from build123d import *

# Parameters (mm, degrees)
BOSS_EXTRUDE1_DEPTH = 1.2
SKETCH1_4_W         = 11
SKETCH1_4_H         = 2.5
BOSS_EXTRUDE2_DEPTH = 1.2
CUT_EXTRUDE1_DEPTH  = 14.654303351
SKETCH4_R           = 6.05
SKETCH4_R_2         = 2.55
CUT_EXTRUDE3_DEPTH  = 0.2


with BuildPart() as part:
    # Sketch1 → Boss-Extrude1 (new body)
    with BuildSketch(Plane(origin=(0, 0, 0), x_dir=(1, 0, 0), z_dir=(0, 1, 0))):
        with BuildLine():
            Line((-5.5, 0), (-1.5, 0))
            ThreePointArc((-1.5, 0), (0, 1.5), (1.5, 0))
            Line((1.5, 0), (5.5, 0))
            Line((5.5, 0), (5.5, 5.5))
            Line((5.5, 5.5), (-5.5, 5.5))
            Line((-5.5, 5.5), (-5.5, 0))
        make_face()
        with BuildLine():
            ThreePointArc((1.5, 0), (0, -1.5), (-1.5, 0))
            Line((-1.5, 0), (-5.5, 0))
            Line((-5.5, 0), (-5.5, -5.5))
            Line((-5.5, -5.5), (5.5, -5.5))
            Line((5.5, -5.5), (5.5, 0))
            Line((5.5, 0), (1.5, 0))
        make_face()
    extrude(amount=BOSS_EXTRUDE1_DEPTH)

    # Sketch1_4 → Boss-Extrude2 (add)
    with BuildSketch(Plane(origin=(0, 0, 0), x_dir=(1, 0, 0), z_dir=(0, 1, 0))):
        with Locations((0, 6.75)):
            Rectangle(SKETCH1_4_W, SKETCH1_4_H)
    extrude(amount=BOSS_EXTRUDE2_DEPTH)

    # Sketch3 → Cut-Extrude1 (cut, through all)
    with BuildSketch(Plane(origin=(5.5, 0, 0), x_dir=(0, 0, -1), z_dir=(1, 0, 0))):
        with BuildLine():
            Line((8, 1.2), (5.5, 1.2))
            add(Edge.make_bspline(
                [(5.5, 1.2), (6.993685342, 0.880481124), (8, 0)],
                knots=[0, 0, 0, 0.506360877, 0.506360877, 0.506360877], degree=2))
            Line((8, 0), (8, 1.2))
        make_face()
    extrude(amount=-CUT_EXTRUDE1_DEPTH, mode=Mode.SUBTRACT)

    # Sketch4 → Cut-Extrude3 (cut)
    with BuildSketch(Plane(origin=(0, 1.2, 0), x_dir=(1, 0, 0), z_dir=(0, 1, 0))):
        Circle(SKETCH4_R)
        with Locations(Location((0, 0, 0), (0, 0, 270))):
            Circle(SKETCH4_R_2, mode=Mode.SUBTRACT)
    extrude(amount=-CUT_EXTRUDE3_DEPTH, mode=Mode.SUBTRACT)


solid = part.part
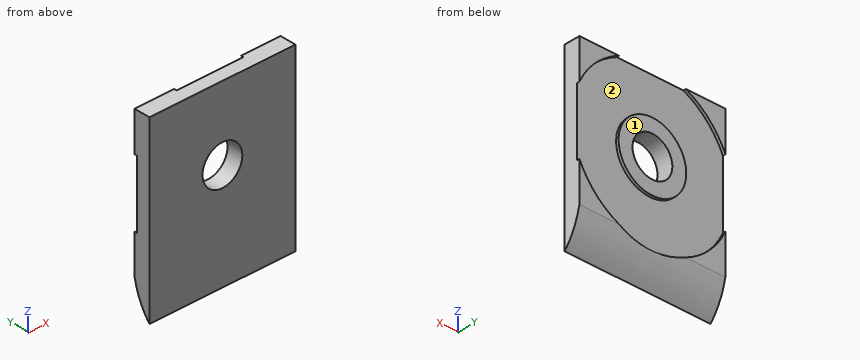
Verification items for the finished model (mm, model axes). Face numbers are marked on the shaded views. Round coordinates to 2 decimals unless told otherwise and drop trailing zeros. Loops run counter-clockwise (first coordinate to the right, second up) from the corner with the lowest first, then second, coordinate; pieces in that order, holes last. Notation, with made-up numbers: (43.25, 65.25) - (73.25, 65.25) arc R26 cw to (73.25, 84.25) - close; hole circle Ø6 at (-23.5, 72). An arc over 180 degrees is marked (long way). Answer in a Markdown table with one row per item. Add a question column.
Q1. Release check for a two-part mould opening along Z. For the marked faces 1 and 2 record: pulls with the +Z half, pulls with the -Z half, needs draft (parallel to the pull), parting line crosses it, or undercut.
Q2. Section check B-B on z = 2.25. Enter the section's corners in (x, y).
Q3. Section check A-A on z = 0. Enter the section's corners in (x, y).
Q4. Material ranges on line 1 (Y direction, x = -3.75, z = -1); line 2 (Z direction, x = 0, y = 0.35); line 3 (Z direction, x = -1.25, y = 0.75), recorded low to high.
Q5. Section check C-C on z = -4.25. Enter the section's corners in (x, y), plus the area to 3 significant figures.
Q6. Gauge pin test, flat end, axial feed: pin 1 (2.5 mm diameter, centred on x = 0, z = 0, fed in from -Y). Record the tip position at first contact, or that the pin passes through.
Found:
| question | item | result |
|---|---|---|
| 1 | face 1 | needs draft |
| 1 | face 2 | undercut |
| 2 | outline | (-5.5, 0) - (5.5, 0) - (5.5, 1) - (1.2, 1) - (1.2, 1.2) - (-1.2, 1.2) - (-1.2, 1) - (-5.5, 1) - close |
| 3 | outline | (-5.5, 0) - (-1.5, 0) - (-1.5, 1.2) - (-2.55, 1.2) - (-2.55, 1) - (-5.5, 1) - close; (1.5, 0) - (5.5, 0) - (5.5, 1) - (2.55, 1) - (2.55, 1.2) - (1.5, 1.2) - close |
| 4 | line 1 | y = 0 to 1 |
| 4 | line 2 | z = -7.55 to -1.5, 1.5 to 5.5 |
| 4 | line 3 | z = -6.85 to -0.83, 0.83 to 5.5 |
| 5 | outline | (-5.5, 0) - (5.5, 0) - (5.5, 1.2) - (4.31, 1.2) - (4.31, 1) - (-4.31, 1) - (-4.31, 1.2) - (-5.5, 1.2) - close |
| 5 | area | 11.5 mm² |
| 6 | pin 1 | passes through |
